Model file for the job. Use its own axes, mm. Round coordinates to 2 decimals unless told otherwise and drop trailing zeros. Loops run counter-clockwise (first coordinate to the right, second up) from the corner with the lowest first, then second, coordinate; pieces in that order, holes last. Notation, with made-up numbers: (77.5, 66.25) -> (101.5, 66.25) arc R6 ccw to (101.5, 75.25) -> close; hole circle Ø8 at (47, 27.25). An arc over 180 degrees is marked (long way). Use a Markdown table: item, result.
from build123d import *

# Parameters (mm, degrees)
SKETCH1_R           = 20
BOSS_EXTRUDE1_DEPTH = 60
SKETCH2_R           = 3.05
CUT_EXTRUDE1_DEPTH  = 30
SKETCH3_R           = 3.29
CUT_EXTRUDE2_DEPTH  = 30
CUT_EXTRUDE3_START  = -100
SKETCH7_R           = 3.05
CUT_EXTRUDE3_DEPTH  = 100


with BuildPart() as part:
    # Sketch1 → Boss-Extrude1 (new body)
    with BuildSketch(Plane.XY):
        Circle(SKETCH1_R)
    extrude(amount=BOSS_EXTRUDE1_DEPTH)

    # Sketch2 → Cut-Extrude1 (cut)
    with BuildSketch(Plane.XY.offset(60)):
        Circle(SKETCH2_R)
    extrude(amount=-CUT_EXTRUDE1_DEPTH, mode=Mode.SUBTRACT)

    # Sketch3 → Cut-Extrude2 (cut)
    with BuildSketch(Plane(origin=(0, 0, 0), x_dir=(-1, 0, 0), z_dir=(0, 0, -1))):
        Circle(SKETCH3_R)
    extrude(amount=-CUT_EXTRUDE2_DEPTH, mode=Mode.SUBTRACT)

    # Sketch6 → Revolve1 (revolve)
    with BuildSketch(Plane(origin=(0, 0, 0), x_dir=(0, 0, -1), z_dir=(1, 0, 0)), mode=Mode.PRIVATE) as revolve1_sk:
        Polygon((-60, 19.998024712), (-80, 0), (-60, 0), align=None)
    revolve(revolve1_sk.sketch.rotate(Axis((0, 0, 60), (0, 0, 1)), 90), axis=Axis((0, 0, 60), (0, 0, 1)))

    # Sketch7 → Cut-Extrude3 (cut)
    with BuildSketch(Plane(origin=(0, 0, 0), x_dir=(-1, 0, 0), z_dir=(0, 0, -1)).offset(CUT_EXTRUDE3_START)):
        with Locations(Location((0, 0, 0), (0, 0, 180))):
            Circle(SKETCH7_R)
    extrude(amount=CUT_EXTRUDE3_DEPTH, mode=Mode.SUBTRACT)


solid = part.part
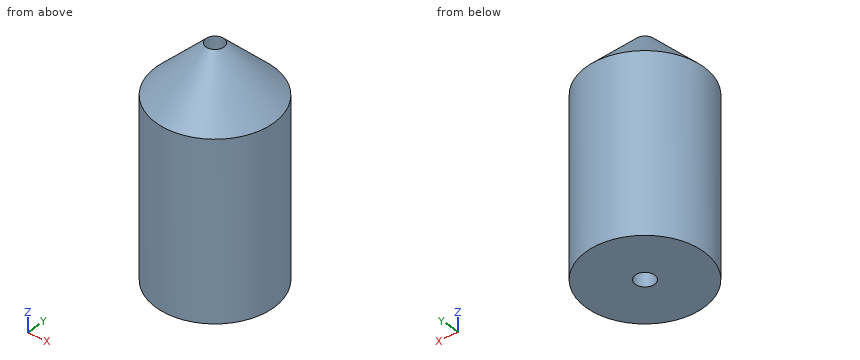
Q1. Band-saw the part on C-C, the plane z = 63.5. Give the cut face in (x, y), plus the area to 3 significant figures.
Results list:
| item | result |
|---|---|
| outline | circle Ø33 at (0, 0); hole circle Ø6.1 at (0, 0) |
| area | 826 mm² |
Q2. Drill centre lines: L1, parallel to Y at x = 0, z = 15.75; L2, parallel to Y at x = 0, z = 61; L3, parallel to X at y = 0.5, z = 22. Where is each one in solid material? Low to high. Write a range as from..to.
Results list:
| item | result |
|---|---|
| L1 | y = -20..-3.29, 3.29..20 |
| L2 | y = -19..-3.05, 3.05..19 |
| L3 | x = -19.99..-3.25, 3.25..19.99 |
Q3. Band-saw the part on B-B, the plane z = 48. Give the cut face in (x, y).
Results list:
| item | result |
|---|---|
| outline | circle Ø40 at (0, 0); hole circle Ø6.1 at (0, 0) |
Q4. Flat gauge pins, fed straight in: pin 1 (2 mm diameter, centred on x = -13, y = 14, fed in from +Z); pin 2 (2 mm diameter, centred on x = 1, y = 1.5, fed in from -Z); pin 3 (6 mm diameter, centred on y = -4.5, z = 63.5, fed in from -X); pin 4 (3 mm diameter, centred on y = -6, z = 58.5, fed in from -X). Where does each tip first touch, or does it go through?
Results list:
| item | result |
|---|---|
| pin 1 | stops at z = 61.89 |
| pin 2 | passes through |
| pin 3 | stops at x = -19.04 |
| pin 4 | stops at x = -19.49 |
